CAD build for the part. Positions are in the model's coordinates, mm. Face numbers are marked on the shaded views. A direction names the side the tool comes from. Give positions to 0.01 mm unless a question says otherwise; leave off trailing zeros. Write each loop counter-clockwise with the first axis right and the second up, starting at its lowest first coordinate (ties: lowest second). Pieces come first, ordered by that corner, then holes. Notation, with made-up numbers: (16.5, 17) - (48.5, 17) arc R25 cw to (48.5, 56) - close; hole circle Ø2 at (74, -17.5). An arc over 180 degrees is marked (long way). Put each result on its own line as item: value. Start each with the question number.
1. Cut at B-B on z = 8. List the corners of the cut face in (x, y).
2. Tool access for the marked faces 5, 6 and 7: list every direction of +Z, -Z, +X, -X, +Y, -Y with a clear straight run to the whole face (end or side of a thin tool).
3. Cut at D-D on y = 3.2. List the corners of the cut face in (x, z) (1 decimal).
4. Mould opens along Z. For the marked faces 1, 2, 3 and 4 say: +Z half, -Z half, draft (parallel to the pull), parting line (faces both ways), or undercut.
5. Cut at A-A on x = 19.5. List the corners of the cut face in (y, z), and give its area (3 significant figures).
6. Drop flat-ended pins along their axis: pin 1 (1.9 mm diameter, centred on x = 3.5, z = 7, fed in from +Y); pin 2 (0.5 mm diameter, centred on x = 2.5, y = 2, fed in from +Z). Give the stop position or say it passes through.
7. Cut at C-C on x = 12.5. List the corners of the cut face in (y, z) (3 decimals).
8. Wall check: line 1 (Z direction, x = 5.5, y = 2.1); line 2 (Z direction, x = 13, y = 3.65) (3 decimals); line 3 (X direction, y = 2.2, z = 11.5). Give the ranges that are in metal, low to high.
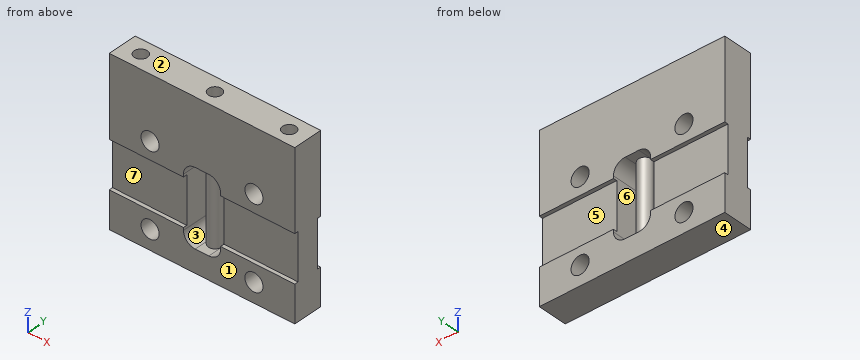
from build123d import *

# Parameters (mm, degrees)
ESBO_O1_W                     = 25
ESBO_O1_H                     = 22
RESSALTO_EXTRUS_O1_DEPTH      = 4
ESBO_O2_W                     = 5
ESBO_O2_H                     = 10.175
CORTE_EXTRUS_O1_DEPTH         = 5
CORTE_EXTRUS_O2_REACH         = 27
ESBO_O3_W                     = 6.3
ESBO_O3_H                     = 0.508
ESBO_O4_W                     = 6.3
ESBO_O4_H                     = 0.508
CORTE_EXTRUS_O3_DEPTH         = 11
ESBO_O5_W                     = 6.35
ESBO_O5_H                     = 0.508
CORTE_EXTRUS_O4_DEPTH         = 11
ESBO_O6_W                     = 6.35
ESBO_O6_H                     = 0.508
CORTE_EXTRUS_O5_DEPTH         = 26
FURO_COM_FOLGA_DE_M21_D       = 2.4384
FURO_COM_FOLGA_DE_M21_DEPTH   = 4
FURO_COM_FOLGA_DE_M1_61_D     = 1.778
FURO_COM_FOLGA_DE_M1_61_DEPTH = 22
FURO_COM_FOLGA_DE_M1_62_D     = 1.778
FURO_COM_FOLGA_DE_M1_62_DEPTH = 3.035
FURO_COM_FOLGA_DE_M1_63_D     = 1.778
FURO_COM_FOLGA_DE_M1_63_DEPTH = 22
FILETE1_R                     = 1.5875
ESBO_O15_R                    = 0.889
RESSALTO_EXTRUS_O2_DEPTH      = 16


with BuildPart() as part:
    # Esboço1 → Ressalto-extrusão1 (new body)
    with BuildSketch(Plane.XZ):
        with Locations((12.5, 11)):
            Rectangle(ESBO_O1_W, ESBO_O1_H)
    extrude(amount=-RESSALTO_EXTRUS_O1_DEPTH)

    # Esboço2 → Corte-extrusão1 (cut, through all)
    with BuildSketch(Plane.XZ):
        with Locations((12.5, 8.1225)):
            Rectangle(ESBO_O2_W, ESBO_O2_H)
    extrude(amount=-CORTE_EXTRUS_O1_DEPTH, mode=Mode.SUBTRACT)

    # Esboço3 → Corte-extrusão2 (cut, up to next)
    with BuildSketch(Plane(origin=(25, 0, 0), x_dir=(0, 0, -1), z_dir=(1, 0, 0)), mode=Mode.PRIVATE) as corte_extrus_o2_sk1:
        with Locations((-8.1225, 0.254)):
            Rectangle(ESBO_O3_W, ESBO_O3_H)
    corte_extrus_o2_tool1 = extrude(corte_extrus_o2_sk1.sketch, amount=-CORTE_EXTRUS_O2_REACH, mode=Mode.PRIVATE) & part.part
    add(corte_extrus_o2_tool1.solids().sort_by_distance((25, 0.254, 8.1225))[0], mode=Mode.SUBTRACT)

    # Esboço4 → Corte-extrusão3 (cut, through all)
    with BuildSketch(Plane(origin=(10, 0, 0), x_dir=(0, 0, -1), z_dir=(1, 0, 0))):
        with Locations((-8.1225, 0.254)):
            Rectangle(ESBO_O4_W, ESBO_O4_H)
    extrude(amount=-CORTE_EXTRUS_O3_DEPTH, mode=Mode.SUBTRACT)

    # Esboço5 → Corte-extrusão4 (cut, through all)
    with BuildSketch(Plane(origin=(10, 0, 0), x_dir=(0, 0, -1), z_dir=(1, 0, 0))):
        with Locations((-8.1225, 3.746)):
            Rectangle(ESBO_O5_W, ESBO_O5_H)
    extrude(amount=-CORTE_EXTRUS_O4_DEPTH, mode=Mode.SUBTRACT)

    # Esboço6 → Corte-extrusão5 (cut, through all)
    with BuildSketch(Plane(origin=(25, 0, 0), x_dir=(0, 0, -1), z_dir=(1, 0, 0))):
        with Locations((-8.1225, 3.746)):
            Rectangle(ESBO_O6_W, ESBO_O6_H)
    extrude(amount=-CORTE_EXTRUS_O5_DEPTH, mode=Mode.SUBTRACT)

    # Furo com folga de M21
    with Locations(Plane(origin=(0, 0, 0), x_dir=(-1, 0, 0), z_dir=(0, -1, 0))):
        with Locations((-19.5, -13.6225), (-19.5, -2.6225), (-5.5, -2.6225), (-5.5, -13.6225)):
            Hole(FURO_COM_FOLGA_DE_M21_D / 2, depth=FURO_COM_FOLGA_DE_M21_DEPTH)

    # Furo com folga de M1.61
    with Locations(Plane(origin=(0, 0, 0), x_dir=(-1, 0, 0), z_dir=(0, 0, -1))):
        with Locations((-2.5, 2), (-22.5, 2)):
            Hole(FURO_COM_FOLGA_DE_M1_61_D / 2, depth=FURO_COM_FOLGA_DE_M1_61_DEPTH)

    # Furo com folga de M1.62
    with Locations(Plane(origin=(0, 0, 0), x_dir=(-1, 0, 0), z_dir=(0, 0, -1))):
        with Locations((-12.5, 2)):
            Hole(FURO_COM_FOLGA_DE_M1_62_D / 2, depth=FURO_COM_FOLGA_DE_M1_62_DEPTH)

    # Furo com folga de M1.63
    with Locations(Plane.XY.offset(22)):
        with Locations((12.5, 2)):
            Hole(FURO_COM_FOLGA_DE_M1_63_D / 2, depth=FURO_COM_FOLGA_DE_M1_63_DEPTH)

    # Filete1
    filete1_edges = [part.edges().sort_by_distance(p)[0] for p in [
        (10, 2, 13.21),
        (15, 2, 13.21),
        (15, 2, 3.035),
        (10, 2, 3.035),
    ]]
    fillet(filete1_edges, radius=FILETE1_R)

    # Esboço15 → Ressalto-extrusão2 (add)
    with BuildSketch(Plane(origin=(0, 0, 0), x_dir=(-1, 0, 0), z_dir=(0, 0, -1))):
        with Locations((-2.5, 2)):
            Circle(ESBO_O15_R)
        with Locations((-12.5, 2)):
            Circle(ESBO_O15_R)
        with Locations((-22.5, 2)):
            Circle(ESBO_O15_R)
    extrude(amount=-RESSALTO_EXTRUS_O2_DEPTH)


solid = part.part
Report:
1. outline: (0, 0.51) - (10, 0.51) - (10, 3.49) - (0, 3.49) - close; circle Ø1.78 at (12.5, 2); (15, 0.51) - (25, 0.51) - (25, 3.49) - (15, 3.49) - close
2. face 5: +X, -X, +Y
2. face 6: +Y, -Y
2. face 7: +X, -X, -Y
3. outline: (0, 0) - (25, 0) - (25, 22) - (0, 22) - close; hole circle Ø2.4 at (5.5, 2.6); hole circle Ø2.4 at (5.5, 13.6); hole (10, 4.6) arc R1.6 ccw to (11.6, 3) - (13.4, 3) arc R1.6 ccw to (15, 4.6) - (15, 11.6) arc R1.6 ccw to (13.4, 13.2) - (11.6, 13.2) arc R1.6 ccw to (10, 11.6) - close; hole circle Ø2.4 at (19.5, 2.6); hole circle Ø2.4 at (19.5, 13.6)
4. face 1: draft
4. face 2: +Z half
4. face 3: undercut
4. face 4: -Z half
5. outline: (0, 0) - (4, 0) - (4, 1.4) - (0, 1.4) - close; (0, 3.84) - (4, 3.84) - (4, 4.95) - (3.49, 4.95) - (3.49, 11.3) - (4, 11.3) - (4, 12.4) - (0, 12.4) - (0, 11.27) - (0.51, 11.27) - (0.51, 4.97) - (0, 4.97) - close; (0, 14.84) - (4, 14.84) - (4, 22) - (0, 22) - close
5. area: 62.1 mm²
6. pin 1: stops at y = 3.49
6. pin 2: stops at z = 16
7. outline: (0, 0) - (4, 0) - (4, 3.035) - (2.889, 3.035) - (2.889, 13.21) - (4, 13.21) - (4, 22) - (2.889, 22) - (2.889, 16) - (1.111, 16) - (1.111, 22) - (0, 22) - (0, 13.21) - (1.111, 13.21) - (1.111, 3.035) - (0, 3.035) - close
8. line 1: z = 0 to 1.4, 3.84 to 12.4, 14.84 to 22
8. line 2: z = 0 to 3.035, 13.21 to 22
8. line 3: x = 0 to 10, 11.63 to 13.37, 15 to 25
